Read the model definition and answer for the solid it produces. Units are mm, in the model's axes. A direction names the side the tool comes from. Give positions to 0.01 mm unless a question says otherwise; leave off trailing zeros. Order: outer loops, then holes, each group sorted by start corner. A loop starts at its lowest first (then second) coordinate and runs counter-clockwise, first axis right, second up. Notation, with made-up numbers: (78, -14) -> (105, -14) arc R18 cw to (105, -6) -> close; hole circle Ø4 at (69, 83.25). An arc over 180 degrees is marked (long way). One line per item, written item: value. Start each with the question number.
from build123d import *

# Parameters (mm, degrees)
BOX_W         = 10
BOX_H         = 10
BOX_DEPTH     = 10
SKETCH_R      = 2.991239
SKETCH_R_2    = 1.537038
PAD_DEPTH     = 0.25
SKETCH001_R   = 3.024278
SKETCH001_R_2 = 1.519206
PAD001_DEPTH  = 0.25
SKETCH002_R   = 3.023334
SKETCH002_R_2 = 1.513555
PAD002_DEPTH  = 0.25
SKETCH003_R   = 3.023333
SKETCH003_R_2 = 1.513555
PAD003_DEPTH  = 0.25
SKETCH004_R   = 2.956459
POCKET_DEPTH  = 1


with BuildPart() as part:
    # Box → Box (new body)
    with BuildSketch(Plane.XY):
        with Locations((5, 5)):
            Rectangle(BOX_W, BOX_H)
    extrude(amount=BOX_DEPTH)

    # Sketch → Pad (new body)
    with BuildSketch(Plane.XY.offset(10)):
        with Locations((5.01728, 5.037612)):
            Circle(SKETCH_R)
        with Locations((5.01728, 5.037612)):
            Circle(SKETCH_R_2, mode=Mode.SUBTRACT)
    extrude(amount=PAD_DEPTH)

    # Sketch001 → Pad001 (new body)
    with BuildSketch(Plane(origin=(0, 0, 0), x_dir=(1, 0, 0), z_dir=(0, 0, -1))):
        with Locations((4.987519, -5.042684)):
            Circle(SKETCH001_R)
        with Locations((4.987519, -5.042684)):
            Circle(SKETCH001_R_2, mode=Mode.SUBTRACT)
    extrude(amount=PAD001_DEPTH)

    # Sketch002 → Pad002 (new body)
    with BuildSketch(Plane.YZ.offset(10)):
        with Locations((5.010271, 4.975845)):
            Circle(SKETCH002_R)
        with Locations((5.010271, 4.975845)):
            Circle(SKETCH002_R_2, mode=Mode.SUBTRACT)
    extrude(amount=PAD002_DEPTH)

    # Sketch003 → Pad003 (new body)
    with BuildSketch(Plane(origin=(0, 0, 0), x_dir=(0, -1, 0), z_dir=(-1, 0, 0))):
        with Locations((-5.010272, 4.975843)):
            Circle(SKETCH003_R)
        with Locations((-5.010272, 4.975843)):
            Circle(SKETCH003_R_2, mode=Mode.SUBTRACT)
    extrude(amount=PAD003_DEPTH)

    # Sketch004 → Pocket (cut)
    with BuildSketch(Plane.XZ):
        with Locations((5.015462, 4.975839)):
            Circle(SKETCH004_R)
    extrude(amount=-POCKET_DEPTH, mode=Mode.SUBTRACT)


solid = part.part
Item 1: Find section B-B on z = 4. Write down the section's boundary in (x, y), then the cut area to 3 significant figures.
Item 2: Find section A-A on x = 5.75. Write down the section's boundary in (y, z), then the cut area to 3 significant figures.
Item 3: Flat-ended cylindrical pins translate along their axes: pin 1 (3 mm diameter, centred on x = 5.02, y = 5.04, fed in from +Z); pin 2 (3.5 mm diameter, centred on x = 5.02, z = 4.98, fed in from -Y); pin 3 (0.9 mm diameter, centred on y = 5.5, z = 5, fed in from -X). Find the tip coordinate at first contact, or state that the pin passes through.
Item 4: For a pull along Z with two mould halves and no side action, classify faces 6 (the flat face through (10, 2.7, 2.7)), 7 (the cylindrical face through (4.37, 0.49, 2.09)), 8 (the flat face through (5, 5, 0)), 9 (the flat face through (5, 5, 10)) as +Z half, -Z half, draft (parallel to the pull), parting line (faces both ways), or undercut.
Item 5: Find the intervals of material crossed by line 1 (Z direction, x = 0.5, y = 1); line 2 (Y direction, x = 6.75, z = 3), in increasing order. Write a range as from..to.
Item 6: Find section C-C on y = 3.25. Write down the section's boundary in (x, z).
Item 7: Find section D-D on x = 2.5. Write down the section's boundary in (y, z).
Item 8: A tool of negligible diameter and unlimited length cuts with its end or side. For faces 1 (the flat face through (2.7, 7.3, 0)), 2 (the flat face through (5, 1, 5)), 3 (the flat face through (5, 10, 5)), 4 (the flat face through (0, 5, 5)), 5 (the flat face through (10, 5, 5)), from which of +Z, -Z, +X, -X, +Y, -Y can it reach the whole face along a straight path? Write none if from no direction.
Checks:
1. outline: (-0.25, 2.15) -> (0, 2.15) -> (0, 0) -> (2.22, 0) -> (2.22, 1) -> (7.81, 1) -> (7.81, 0) -> (10, 0) -> (10, 2.15) -> (10.25, 2.15) -> (10.25, 3.85) -> (10, 3.85) -> (10, 6.17) -> (10.25, 6.17) -> (10.25, 7.87) -> (10, 7.87) -> (10, 10) -> (0, 10) -> (0, 7.87) -> (-0.25, 7.87) -> (-0.25, 6.17) -> (0, 6.17) -> (0, 3.85) -> (-0.25, 3.85) -> close
1. area: 96.1 mm2
2. outline: (0, 0) -> (2.12, 0) -> (2.12, -0.25) -> (3.73, -0.25) -> (3.73, 0) -> (6.36, 0) -> (6.36, -0.25) -> (7.97, -0.25) -> (7.97, 0) -> (10, 0) -> (10, 10) -> (7.94, 10) -> (7.94, 10.25) -> (6.39, 10.25) -> (6.39, 10) -> (3.69, 10) -> (3.69, 10.25) -> (2.14, 10.25) -> (2.14, 10) -> (0, 10) -> (0, 7.84) -> (1, 7.84) -> (1, 2.11) -> (0, 2.11) -> close
2. area: 95.9 mm2
3. pin 1: z = 10
3. pin 2: y = 1
3. pin 3: x = 0
4. face 6: draft
4. face 7: undercut
4. face 8: -Z half
4. face 9: +Z half
5. line 1: 0..10
5. line 2: 1..10
6. outline: (-0.25, 2.52) -> (0, 2.52) -> (0, 0) -> (2.55, 0) -> (2.55, -0.25) -> (7.42, -0.25) -> (7.42, 0) -> (10, 0) -> (10, 2.52) -> (10.25, 2.52) -> (10.25, 7.43) -> (10, 7.43) -> (10, 10) -> (7.42, 10) -> (7.42, 10.25) -> (2.62, 10.25) -> (2.62, 10) -> (0, 10) -> (0, 7.43) -> (-0.25, 7.43) -> close
7. outline: (0, 0) -> (3.32, 0) -> (3.32, -0.25) -> (6.76, -0.25) -> (6.76, 0) -> (10, 0) -> (10, 10) -> (6.65, 10) -> (6.65, 10.25) -> (3.42, 10.25) -> (3.42, 10) -> (0, 10) -> (0, 6.53) -> (1, 6.53) -> (1, 3.42) -> (0, 3.42) -> close
8. face 1: -Z
8. face 2: -Y
8. face 3: +Z, -Z, +X, -X, +Y
8. face 4: -X
8. face 5: +X
